Design review of the part shown in the three views and the two pictorial views. Dimensions are in mm from the part's minimum x, y and z. Coordinates: 2 decimals unless noted, no trailing zeros. Loops run counter-clockwise (first coordinate to the right, second up) from the corner with the lowest first, then second, coordinate; pieces in that order, holes last. Notation, with made-up numbers: (-31, 9) -> (-4, 9) arc R6 ccw to (-4, 20) -> close; hole circle Ø3 at (66, 46). An arc over 180 degrees is marked (long way). Answer in a Markdown table with one row per item.
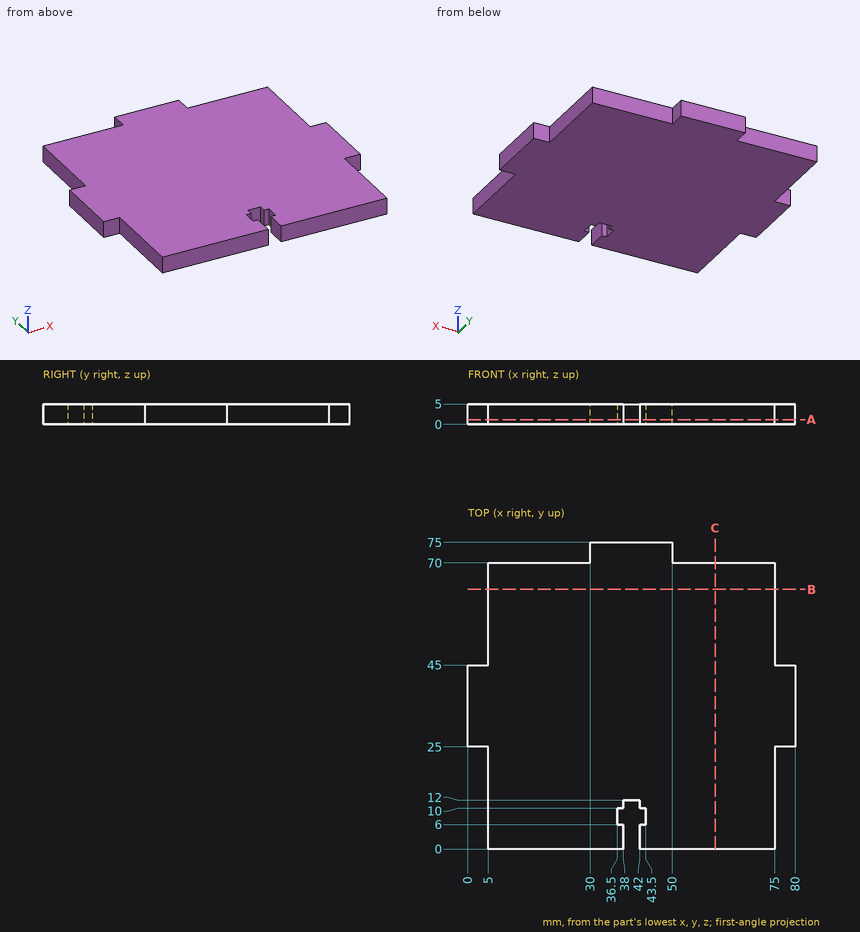
Item 1: Insertion check: pin 1 (1.5 mm diameter, centred on y = 73.5, z = 2.5, fed in from +X); pin 2 (2 mm diameter, centred on y = 11, z = 1.5, fed in from -X); pin 3 (2.5 mm diameter, centred on y = 60.5, z = 3.5, fed in from +X); pin 4 (1.6 mm diameter, centred on x = 43, z = 2.5, fed in from -Y). Each pin has a flat end and moves straight along its axis. Give the tip position at first contact, or say it passes through.
Worked answers:
| item | result |
|---|---|
| pin 1 | x = 50 |
| pin 2 | x = 5 |
| pin 3 | x = 75 |
| pin 4 | y = 0 |
Item 2: Take a section at B-B, the plane y = 63.5. State the section outline as (x, z) points, and give its area (3 significant figures).
Worked answers:
| item | result |
|---|---|
| outline | (5, 0) -> (75, 0) -> (75, 5) -> (5, 5) -> close |
| area | 350 mm² |
Item 3: Take a section at C-C, the plane x = 60.5. State the section outline as (y, z) points.
Worked answers:
| item | result |
|---|---|
| outline | (0, 0) -> (70, 0) -> (70, 5) -> (0, 5) -> close |
Item 4: For L1, parallel to X at y = 6.5, z = 1.6; L2, parallel to Y at x = 58.5, z = 3.2; L3, parallel to X at y = 5.5, z = 3.5, list the stretches that pass through material, from the lowest coordinate up.
Worked answers:
| item | result |
|---|---|
| L1 | 5 to 36.5, 43.5 to 75 |
| L2 | 0 to 70 |
| L3 | 5 to 38, 42 to 75 |
Item 5: Take a section at A-A, the plane z = 1.2. State the section outline as (x, y) points.
Worked answers:
| item | result |
|---|---|
| outline | (0, 25) -> (5, 25) -> (5, 0) -> (38, 0) -> (38, 6) -> (36.5, 6) -> (36.5, 10) -> (38, 10) -> (38, 12) -> (42, 12) -> (42, 10) -> (43.5, 10) -> (43.5, 6) -> (42, 6) -> (42, 0) -> (75, 0) -> (75, 25) -> (80, 25) -> (80, 45) -> (75, 45) -> (75, 70) -> (50, 70) -> (50, 75) -> (30, 75) -> (30, 70) -> (5, 70) -> (5, 45) -> (0, 45) -> close |
